Autodesk Inventor part; units mm, degrees
ref_plane "YZ Plane" through (0, 0, 0) normal (1, 0, 0) x (0, 1, 0)
ref_plane "XZ Plane" through (0, 0, 0) normal (0, 1, 0) x (-1, 0, 0)
ref_plane "XY Plane" through (0, 0, 0) normal (0, 0, 1) x (1, 0, 0)
sketch "Sketch1" plane through (0, 0, 0) normal (0, 1, 0) x (-1, 0, 0)
  arc A0 (1.4918, 12.1563) -> (-1.4918, 12.1563) centre (0, 12) ccw
  arc A1 (-1.4918, -12.1563) -> (1.4918, -12.1563) centre (0, -12) ccw
  line L0 (0, -12) -> (0, 12) construction
  line L1 (-2.735, 0.2865) -> (-1.4918, 12.1563)
  line L2 (1.4918, -12.1563) -> (2.735, -0.2865)
  line L3 (-1.4918, -12.1563) -> (-2.735, -0.2865)
  line L4 (2.735, 0.2865) -> (1.4918, 12.1563)
  arc A2 (-2.735, 0.2865) -> (-2.735, -0.2865) centre (0, 0) ccw
  arc A3 (2.735, -0.2865) -> (2.735, 0.2865) centre (0, 0) ccw
  line L5 (2.75, 0) -> (-2.75, 0) construction
  line L6 (-3.0334, -0.3177) -> (-1.7902, -12.1875)
  arc A4 (-1.7902, -12.1875) -> (1.7902, -12.1875) centre (0, -12) ccw
  line L7 (1.7902, -12.1875) -> (3.0334, -0.3177)
  arc A5 (3.0334, -0.3177) -> (3.0334, 0.3177) centre (0, 0) ccw
  line L8 (3.0334, 0.3177) -> (1.7902, 12.1875)
  arc A6 (1.7902, 12.1875) -> (-1.7902, 12.1875) centre (0, 12) ccw
  line L9 (-1.7902, 12.1875) -> (-3.0334, 0.3177)
  arc A7 (-3.0334, 0.3177) -> (-3.0334, -0.3177) centre (0, 0) ccw
  line L10 (0, -4.275) -> (0, 57.15) construction
  line L11 (-6.35, -10.625) -> (-6.35, 50.8)
  line L12 (6.35, 50.8) -> (6.35, -10.625)
  arc A8 (-6.35, -10.625) -> (6.35, -10.625) centre (0, -10.625) ccw
  arc A9 (6.35, 50.8) -> (-6.35, 50.8) centre (0, 50.8) ccw
  circle A10 centre (0, 50.8) radius 1.5875
  point P0 (0, 0)
  point P1 (0, -13.8)
  point P2 (0, -16.975)
  dimension "d5" = 3
  dimension "d6" = 3
  dimension "d7" = 24
  dimension "d8" = 5.5
  dimension "d9" = 0.3
  dimension "d13" = 50.8
  dimension "d15" = 3.175
  dimension "d17" = 3.175
  dimension "d19" = 6.35
  dimension "d20" = 6.35
extrude "Extrusion1" add sketch "Sketch1" along normal blind 1.5875 contours L11 A9 L12 A8
sketch "Sketch2" plane through (0, 1.5875, 0) normal (0, 1, 0) x (1, 0, 0)
  line L0 (6.35, -50.8) -> (6.35, 10.625)
  arc A0 (6.35, 10.625) -> (-6.35, 10.625) centre (0, 10.625) ccw
  line L1 (-6.35, 10.625) -> (-6.35, -50.8)
  arc A1 (-6.35, -50.8) -> (6.35, -50.8) centre (0, -50.8) ccw
  arc A2 (3.0334, -0.3177) -> (3.0334, 0.3177) centre (0, 0) ccw
  line L2 (3.0334, -0.3177) -> (1.7902, -12.1875)
  arc A3 (-1.7902, -12.1875) -> (1.7902, -12.1875) centre (0, -12) ccw
  line L3 (-1.7902, -12.1875) -> (-3.0334, -0.3177)
  arc A4 (-3.0334, 0.3177) -> (-3.0334, -0.3177) centre (0, 0) ccw
  line L4 (-3.0334, 0.3177) -> (-1.7902, 12.1875)
  arc A5 (1.7902, 12.1875) -> (-1.7902, 12.1875) centre (0, 12) ccw
  line L5 (1.7902, 12.1875) -> (3.0334, 0.3177)
  circle A6 centre (0, -50.8) radius 1.5875
extrude "Extrusion2" add sketch "Sketch2" along normal blind 1.5875 contours A1 L1 A0 L0 | L2 A3 L3 A4 L4 A5 L5 A2
properties part number "arm3"
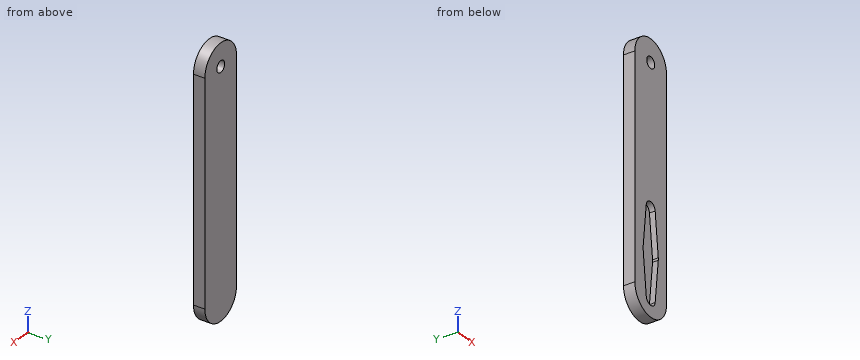
Verification items for the finished model (mm, model axes). Give positions to 0.01 mm unless a question says otherwise; leave off trailing zeros. Loops run counter-clockwise (first coordinate to the right, second up) from the corner with the lowest first, then second, coordinate; pieces in that order, holes last.
1) Thickness scan on line 1 along X through (y, z) = (2.5, 50.8); line 2 along Z through (x, y) = (0.75, 1.3); line 3 along Y through (x, z) = (1.25, 7.5) (1 decimal). Record the ranges inside material, lowest first.
2) Sectioned sample at A-A, the plane y = 0.75. Count the separate pieces of the cut face and the enclosed holes in it, then the cut area to 3 significant figures.
3) Depth check by flat-ended pin: pin 1 Ø3 at (x, z) = (0, 50.8) entering from +Y; pin 2 Ø1 at (x, y) = (1, 1) entering from +Z; pin 3 Ø1.8 at (x, z) = (1, 6.5) entering from -Y. Enter the tip coordinate at first touch or a pass-through.
4) Sectioned sample at C-C, the plane x = -4. Enter the section's corners in (y, z) (3 decimals), then the cut area to 3 significant figures.
Answers:
1. line 1: x = -6.35 to -1.59, 1.59 to 6.35
1. line 2: z = -16.93 to -13.64, 13.64 to 49.4, 52.2 to 57.11
1. line 3: y = 1.6 to 3.2
2. separate pieces: 1
2. enclosed holes: 2
2. area: 772 mm2
3. pin 1: passes through
3. pin 2: stops at z = 57.13
3. pin 3: stops at y = 1.59
4. outline: (0, -15.557) - (3.175, -15.557) - (3.175, 55.732) - (0, 55.732) - close
4. area: 226 mm2
